```python
from build123d import *

# Parameters (mm, degrees)
F1_DEPTH = 2
F2_DEPTH = 8
F3_DEPTH = 7.25


with BuildPart() as f1:
    # F0 (on Top) → F1 (new body)
    with BuildSketch(Plane.XY):
        with BuildLine():
            Line((4.85, 7.2), (-4.85, 7.2))
            ThreePointArc((-4.85, 7.2), (-6.511701, 6.511701), (-7.2, 4.85))
            Line((-7.2, 4.85), (-7.2, -4.85))
            ThreePointArc((-7.2, -4.85), (-6.511701, -6.511701), (-4.85, -7.2))
            Line((-4.85, -7.2), (4.85, -7.2))
            ThreePointArc((4.85, -7.2), (6.511701, -6.511701), (7.2, -4.85))
            Line((7.2, -4.85), (7.2, 4.85))
            ThreePointArc((7.2, 4.85), (6.511701, 6.511701), (4.85, 7.2))
        make_face()
        with BuildLine():
            ThreePointArc((6.45, -4.85), (5.981371, -5.981371), (4.85, -6.45))
            Line((4.85, -6.45), (-4.85, -6.45))
            ThreePointArc((-4.85, -6.45), (-5.981371, -5.981371), (-6.45, -4.85))
            Line((-6.45, -4.85), (-6.45, 4.85))
            ThreePointArc((-6.45, 4.85), (-5.981371, 5.981371), (-4.85, 6.45))
            Line((-4.85, 6.45), (4.85, 6.45))
            ThreePointArc((4.85, 6.45), (5.981371, 5.981371), (6.45, 4.85))
            Line((6.45, 4.85), (6.45, -4.85))
        make_face(mode=Mode.SUBTRACT)
    extrude(amount=F1_DEPTH)

    # F0 (on Top) → F2 (join)
    with BuildSketch(Plane.XY):
        with BuildLine():
            Line((-4.85, -6.45), (4.85, -6.45))
            ThreePointArc((4.85, -6.45), (5.981371, -5.981371), (6.45, -4.85))
            Line((6.45, -4.85), (6.45, 4.85))
            ThreePointArc((6.45, 4.85), (5.981371, 5.981371), (4.85, 6.45))
            Line((4.85, 6.45), (-4.85, 6.45))
            ThreePointArc((-4.85, 6.45), (-5.981371, 5.981371), (-6.45, 4.85))
            Line((-6.45, 4.85), (-6.45, -4.85))
            ThreePointArc((-6.45, -4.85), (-5.981371, -5.981371), (-4.85, -6.45))
        make_face()
        Polygon((-2.438525, -2.531762), (-1.68306, -1.699795), (-1.552468, -1.911373), (-1.404542, -2.096653), (-1.32408, -2.179431), (-1.239284, -2.255635), (-1.150156, -2.325265), (-1.056694, -2.38832), (-0.959721, -2.444352), (-0.860058, -2.492913), (-0.757706, -2.534004), (-0.652664, -2.567623), (-0.544933, -2.593771), (-0.434512, -2.612449), (-0.321401, -2.623655), (-0.205601, -2.627391), (-0.036384, -2.62048), (0.124616, -2.599748), (0.277397, -2.565195), (0.42196, -2.51682), (0.558306, -2.454625), (0.686433, -2.378607), (0.806342, -2.288769), (0.918033, -2.185109), (1.018891, -2.070168), (1.106301, -1.946487), (1.180264, -1.814064), (1.240779, -1.6729), (1.287846, -1.522995), (1.321465, -1.364349), (1.341637, -1.196961), (1.348361, -1.020833), (1.341301, -0.851541), (1.32012, -0.690318), (1.28482, -0.537163), (1.2354, -0.392077), (1.171859, -0.255059), (1.094198, -0.12611), (1.002417, -0.00523), (0.896516, 0.107582), (0.779185, 0.209561), (0.653112, 0.297942), (0.518299, 0.372727), (0.374744, 0.433914), (0.222448, 0.481504), (0.061411, 0.515497), (-0.108366, 0.535893), (-0.286885, 0.542691), (-0.502796, 0.533278), (-0.710639, 0.505038), (-0.910412, 0.45797), (-1.102117, 0.392077), (-1.28426, 0.307655), (-1.455345, 0.205003), (-1.615373, 0.084123), (-1.764344, -0.054986), (-2.046448, 0.007172), (-1.17623, 3.559768), (2.132514, 3.559768), (2.132514, 2.636954), (-0.492486, 2.636954), (-0.903689, 1.092555), (-0.621585, 1.196551), (-0.349044, 1.269467), (-0.081284, 1.3125), (0.186475, 1.326844), (0.430477, 1.316833), (0.662824, 1.2868), (0.883517, 1.236744), (1.092555, 1.166667), (1.289938, 1.076567), (1.475666, 0.966445), (1.64974, 0.8363), (1.812158, 0.686134), (1.958963, 0.519905), (2.086194, 0.341573), (2.19385, 0.151138), (2.281933, -0.0514), (2.350442, -0.266041), (2.399377, -0.492785), (2.428738, -0.731632), (2.438525, -0.982582), (2.427094, -1.269206), (2.392802, -1.540962), (2.335649, -1.797852), (2.255635, -2.039874), (2.15276, -2.267028), (2.027024, -2.479316), (1.878426, -2.676736), (1.706967, -2.85929), (1.516308, -3.023464), (1.310109, -3.165749), (1.088371, -3.286143), (0.851093, -3.384648), (0.598275, -3.461263), (0.329918, -3.515988), (0.046021, -3.548823), (-0.253415, -3.559768), (-0.432121, -3.555846), (-0.60485, -3.544079), (-0.771602, -3.524467), (-0.932377, -3.497012), (-1.087176, -3.461711), (-1.235997, -3.418566), (-1.378842, -3.367577), (-1.51571, -3.308743), (-1.647274, -3.241691), (-1.774206, -3.166048), (-1.896506, -3.081812), (-2.014173, -2.988986), (-2.127209, -2.887567), (-2.235613, -2.777557), (-2.339385, -2.658956), align=None, mode=Mode.SUBTRACT)
    extrude(amount=F2_DEPTH)

    # F0 (on Top) → F3 (join)
    with BuildSketch(Plane.XY):
        Polygon((-1.552468, -1.911373), (-1.68306, -1.699795), (-2.438525, -2.531762), (-2.339385, -2.658956), (-2.235613, -2.777557), (-2.127209, -2.887567), (-2.014173, -2.988986), (-1.896506, -3.081812), (-1.774206, -3.166048), (-1.647274, -3.241691), (-1.51571, -3.308743), (-1.378842, -3.367577), (-1.235997, -3.418566), (-1.087176, -3.461711), (-0.932377, -3.497012), (-0.771602, -3.524467), (-0.60485, -3.544079), (-0.432121, -3.555846), (-0.253415, -3.559768), (0.046021, -3.548823), (0.329918, -3.515988), (0.598275, -3.461263), (0.851093, -3.384648), (1.088371, -3.286143), (1.310109, -3.165749), (1.516308, -3.023464), (1.706967, -2.85929), (1.878426, -2.676736), (2.027024, -2.479316), (2.15276, -2.267028), (2.255635, -2.039874), (2.335649, -1.797852), (2.392802, -1.540962), (2.427094, -1.269206), (2.438525, -0.982582), (2.428738, -0.731632), (2.399377, -0.492785), (2.350442, -0.266041), (2.281933, -0.0514), (2.19385, 0.151138), (2.086194, 0.341573), (1.958963, 0.519905), (1.812158, 0.686134), (1.64974, 0.8363), (1.475666, 0.966445), (1.289938, 1.076567), (1.092555, 1.166667), (0.883517, 1.236744), (0.662824, 1.2868), (0.430477, 1.316833), (0.186475, 1.326844), (-0.081284, 1.3125), (-0.349044, 1.269467), (-0.621585, 1.196551), (-0.903689, 1.092555), (-0.492486, 2.636954), (2.132514, 2.636954), (2.132514, 3.559768), (-1.17623, 3.559768), (-2.046448, 0.007172), (-1.764344, -0.054986), (-1.615373, 0.084123), (-1.455345, 0.205003), (-1.28426, 0.307655), (-1.102117, 0.392077), (-0.910412, 0.45797), (-0.710639, 0.505038), (-0.502796, 0.533278), (-0.286885, 0.542691), (-0.108366, 0.535893), (0.061411, 0.515497), (0.222448, 0.481504), (0.374744, 0.433914), (0.518299, 0.372727), (0.653112, 0.297942), (0.779185, 0.209561), (0.896516, 0.107582), (1.002417, -0.00523), (1.094198, -0.12611), (1.171859, -0.255059), (1.2354, -0.392077), (1.28482, -0.537163), (1.32012, -0.690318), (1.341301, -0.851541), (1.348361, -1.020833), (1.341637, -1.196961), (1.321465, -1.364349), (1.287846, -1.522995), (1.240779, -1.6729), (1.180264, -1.814064), (1.106301, -1.946487), (1.018891, -2.070168), (0.918033, -2.185109), (0.806342, -2.288769), (0.686433, -2.378607), (0.558306, -2.454625), (0.42196, -2.51682), (0.277397, -2.565195), (0.124616, -2.599748), (-0.036384, -2.62048), (-0.205601, -2.627391), (-0.321401, -2.623655), (-0.434512, -2.612449), (-0.544933, -2.593771), (-0.652664, -2.567623), (-0.757706, -2.534004), (-0.860058, -2.492913), (-0.959721, -2.444352), (-1.056694, -2.38832), (-1.150156, -2.325265), (-1.239284, -2.255635), (-1.32408, -2.179431), (-1.404542, -2.096653), align=None)
    extrude(amount=F3_DEPTH)


solid = f1.part
```
Geometry: final body of the model. Coordinates: model frame, mm. A direction names the side the tool comes from. Coordinates: 2 decimals unless noted, no trailing zeros. Order: outer loops, then holes, each group sorted by start corner. A loop starts at its lowest first (then second) coordinate and runs counter-clockwise, first axis right, second up. Notation, with made-up numbers: M -24.75,75.5 L -16.75,75.5 A18 ccw -16.75,108.5 Z; hole C -20.5,39 d5. An arc over 180 degrees is marked long. Answer in a Markdown table with one row per item. Add a question column.
Q1. Contact query for flat-ended pins moving along their axis: P1, Ø0.6, axis at x = 0.5, z = 7.5, coming from the -Y side; P2, Ø1, axis at x = -2, z = 4.5, coming from the +Y side; P3, Ø3, axis at y = 2, z = 5.5, coming from the -X side. Output: stop coordinate, or through.
Q2. Section query A-A on y = -4.5. Return the cut outline in (x, z), and give its area (3 significant figures).
Q3. Line query: L1, parallel to X at y = 0, z = 7; L2, parallel to Y at x = 0.75, z = 7.5. Output: solid intervals per line, ascending.
Q4. Section query C-C on y = 1.75. Return the cut outline in (x, z), and give its area (3 significant figures).
Q5. Reachability of faces 1 (the cylindrical face through (5.97, -5.99, 4.96)), 2 (the flat face through (0, 6.45, 5)), 3 (the cylindrical face through (-5.97, 5.99, 4.96)) from +Z, -Z, +X, -X, +Y, -Y: full face, straight path, thin tool, end or side. Return the list, or none.
Q6. Mould query, pull axis Y, two halves, no side actions, for faces 4 (the flat face through (0, 1, 7.25)), 5 (the flat face through (6.45, 0, 5)), 6 (the cylindrical face through (5.99, 5.97, 4.96)), 7 (the cylindrical face through (6.493, -6.53, 0.986)). Classes: released by +Y, released by -Y, zero draft, split by the parting line, or undercut.
Completed:
| question | item | result |
|---|---|---|
| 1 | P1 | stops at y = -6.45 |
| 1 | P2 | stops at y = 6.45 |
| 1 | P3 | stops at x = -6.45 |
| 2 | outline | M -7.2,0 L 7.2,0 L 7.2,2 L 6.45,2 L 6.45,8 L -6.45,8 L -6.45,2 L -7.2,2 Z |
| 2 | area | 106 mm2 |
| 3 | L1 | x = -6.45 to 6.45 |
| 3 | L2 | y = -6.45 to -3.42, -2.33 to 0.23, 1.27 to 2.64, 3.56 to 6.45 |
| 4 | outline | M -7.2,0 L 7.2,0 L 7.2,2 L 6.45,2 L 6.45,8 L -0.73,8 L -0.73,7.25 L -1.62,7.25 L -1.62,8 L -6.45,8 L -6.45,2 L -7.2,2 Z |
| 4 | area | 106 mm2 |
| 5 | face 1 | +Z, +X, -Y |
| 5 | face 2 | +Z, +X, -X, +Y |
| 5 | face 3 | +Z, -X, +Y |
| 6 | face 4 | undercut |
| 6 | face 5 | zero draft |
| 6 | face 6 | released by +Y |
| 6 | face 7 | released by -Y |
